Can you work these out from the model? Positions are in its coordinate system, mm. A direction names the side the tool comes from. Round coordinates to 2 decimals unless told otherwise and drop trailing zeros. Write each loop counter-clockwise with the first axis right and the second up, starting at its lowest first coordinate (ties: lowest second). Pieces come first, ordered by that corner, then holes. Notation, with made-up numbers: (8.25, 8) -> (13.25, 8) arc R5 ccw to (13.25, 15) -> close; hole circle Ø4 at (56, -7.5). An arc over 180 degrees is marked (long way). Use CSV: the item, a comma, the result in double quotes.
```python
from build123d import *

# Parameters (mm, degrees)
SKETCH1_R             = 19
BOSS_EXTRUDE1_DEPTH   = 24.3
BOSS_EXTRUDE2_DEPTH   = 4.35
SKETCH2_R             = 15.85
BOSS_EXTRUDE3_DEPTH   = 45
CORTE_EXTRUS_O1_REACH = 71.3
ESBO_O3_R             = 1.5


with BuildPart() as part:
    # Sketch1 → Boss-Extrude1 (new body)
    with BuildSketch(Plane(origin=(0, 0, 0), x_dir=(0, 0, -1), z_dir=(1, 0, 0))):
        Circle(SKETCH1_R)
    extrude(amount=-BOSS_EXTRUDE1_DEPTH)

    # Sketch1_3 → Boss-Extrude2 (add)
    with BuildSketch(Plane(origin=(0, 0, 0), x_dir=(0, 0, -1), z_dir=(1, 0, 0))):
        with BuildLine():
            Line((3.5e-08, 19), (-19, 19))
            Line((-19, 19), (-19, -9e-09))
            ThreePointArc((-19, -9e-09), (-13.435028834, 13.435028851), (3.5e-08, 19))
        make_face()
        with BuildLine():
            Line((19, 19), (3.5e-08, 19))
            ThreePointArc((3.5e-08, 19), (13.435028855, 13.43502883), (19, 0))
            Line((19, 0), (19, 19))
        make_face()
        with BuildLine():
            Line((19, -19), (19, 0))
            ThreePointArc((19, 0), (13.435028852, -13.435028833), (2.8e-08, -19))
            Line((2.8e-08, -19), (19, -19))
        make_face()
        with BuildLine():
            ThreePointArc((2.8e-08, -19), (-13.435028829, -13.435028856), (-19, -9e-09))
            Line((-19, -9e-09), (-19, -19))
            Line((-19, -19), (2.8e-08, -19))
        make_face()
    extrude(amount=-BOSS_EXTRUDE2_DEPTH)

    # Sketch2 → Boss-Extrude3 (add)
    with BuildSketch(Plane.ZY.offset(24.3)):
        Circle(SKETCH2_R)
    extrude(amount=BOSS_EXTRUDE3_DEPTH)

    # Esbo_o2 → Revolu_o1 (revolve)
    with BuildSketch(Plane.XY):
        Polygon((0, -1.2), (6.6, -1.2), (6.6, -4.2), (21.5, -4.2), (21.5, -7.2), (0, -7.2), align=None)
    revolve(axis=Axis((0, -7.2, 0), (1, 0, 0)))

    # Esbo_o3 → Corte-extrus_o1 (cut, up to next)
    with BuildSketch(Plane(origin=(0, 0, 0), x_dir=(0, 0, -1), z_dir=(1, 0, 0)), mode=Mode.PRIVATE) as corte_extrus_o1_sk1:
        with Locations((-16, 16)):
            Circle(ESBO_O3_R)
    corte_extrus_o1_tool1 = extrude(corte_extrus_o1_sk1.sketch, amount=-CORTE_EXTRUS_O1_REACH, mode=Mode.PRIVATE) & part.part
    add(corte_extrus_o1_tool1.solids().sort_by_distance((0, 16, 16))[0], mode=Mode.SUBTRACT)
    # Esbo_o3 → Corte-extrus_o1 (cut, up to next)
    with BuildSketch(Plane(origin=(0, 0, 0), x_dir=(0, 0, -1), z_dir=(1, 0, 0)), mode=Mode.PRIVATE) as corte_extrus_o1_sk2:
        with Locations((16, 16)):
            Circle(ESBO_O3_R)
    corte_extrus_o1_tool2 = extrude(corte_extrus_o1_sk2.sketch, amount=-CORTE_EXTRUS_O1_REACH, mode=Mode.PRIVATE) & part.part
    add(corte_extrus_o1_tool2.solids().sort_by_distance((0, 16, -16))[0], mode=Mode.SUBTRACT)
    # Esbo_o3 → Corte-extrus_o1 (cut, up to next)
    with BuildSketch(Plane(origin=(0, 0, 0), x_dir=(0, 0, -1), z_dir=(1, 0, 0)), mode=Mode.PRIVATE) as corte_extrus_o1_sk3:
        with Locations((-16, -16)):
            Circle(ESBO_O3_R)
    corte_extrus_o1_tool3 = extrude(corte_extrus_o1_sk3.sketch, amount=-CORTE_EXTRUS_O1_REACH, mode=Mode.PRIVATE) & part.part
    add(corte_extrus_o1_tool3.solids().sort_by_distance((0, -16, 16))[0], mode=Mode.SUBTRACT)
    # Esbo_o3 → Corte-extrus_o1 (cut, up to next)
    with BuildSketch(Plane(origin=(0, 0, 0), x_dir=(0, 0, -1), z_dir=(1, 0, 0)), mode=Mode.PRIVATE) as corte_extrus_o1_sk4:
        with Locations((16, -16)):
            Circle(ESBO_O3_R)
    corte_extrus_o1_tool4 = extrude(corte_extrus_o1_sk4.sketch, amount=-CORTE_EXTRUS_O1_REACH, mode=Mode.PRIVATE) & part.part
    add(corte_extrus_o1_tool4.solids().sort_by_distance((0, -16, -16))[0], mode=Mode.SUBTRACT)


solid = part.part
```
Q1. Will these pins go through, and if not, where does the flat tip stop? P1, Ø1, axis at x = -53, y = -9, coming from the -Z side; P2, Ø5, axis at y = -8.5, z = 4, coming from the +X side; P3, Ø4, axis at y = 11, z = -1, coming from the +X side; P4, Ø5, axis at x = -52, y = 3.5, coming from the -Z side.
Resolved:
P1,"stops at z = -13.38"
P2,"stops at x = 21.5"
P3,"stops at x = 0"
P4,"stops at z = -15.82"
Q2. Please list where these lines run through material, in increasing order: probe 1 along Y at (x, z) = (-1.35, 16); probe 2 along X at (y, z) = (3.5, -6.5); probe 3 along Z at (x, y) = (-19.5, 10.5).
Resolved:
probe 1,"y = -19 to -17.5, -14.5 to 14.5, 17.5 to 19"
probe 2,"x = -69.3 to 0"
probe 3,"z = -15.84 to 15.84"
Q3. Suppose I cut it at A-A (z = 11.5). Write out the boundary of the cut face in (x, y), and give its area (3 significant figures).
Resolved:
outline,"(-69.3, -10.91) -> (-24.3, -10.91) -> (-24.3, -15.12) -> (-4.35, -15.12) -> (-4.35, -19) -> (0, -19) -> (0, 19) -> (-4.35, 19) -> (-4.35, 15.12) -> (-24.3, 15.12) -> (-24.3, 10.91) -> (-69.3, 10.91) -> close"
area,"1,750 mm^2"
Q4. Suppose I cut it at B-B (y = -7.2). Write out the boundary of the cut face in (x, z), and give its area (3 significant figures).
Resolved:
outline,"(-69.3, -14.12) -> (-24.3, -14.12) -> (-24.3, -17.58) -> (-4.35, -17.58) -> (-4.35, -19) -> (0, -19) -> (0, -6) -> (6.6, -6) -> (6.6, -3) -> (21.5, -3) -> (21.5, 3) -> (6.6, 3) -> (6.6, 6) -> (0, 6) -> (0, 19) -> (-4.35, 19) -> (-4.35, 17.58) -> (-24.3, 17.58) -> (-24.3, 14.12) -> (-69.3, 14.12) -> close"
area,"2,310 mm^2"
Q5. On a 3-axis mill with a long thin cutter (end or side, diameter ignored), from which of +Z, -Z, +X, -X, +Y, -Y can I reach the whole of each face in a straight line? I mean faces 4 (the face through (-14.185, -16.856, -8.767)), 5 (the face through (-4.35, -14, -14)), 6 (the face through (3.346, -1.477, 1.802)). Say none if no direction works.
Resolved:
face 4,"-X"
face 5,"-Z, -X, -Y"
face 6,"+X"
Q6. If we mould it in two halves opening along Y, with no side actions, what happens to faces 1 (the face through (21.5, -7, 0)), 2 (the face through (-2.14, 16.07, -14.5)), 3 (the face through (-2, -19, 0))? For each: released by +Y, released by -Y, zero draft, split by the parting line, or undercut.
Resolved:
face 1,"zero draft"
face 2,"undercut"
face 3,"released by -Y"
Q7. Suppose I cut it at C-C (x = -8). Write out the boundary of the cut face in (y, z).
Resolved:
outline,"circle Ø38 at (0, 0)"
